Verification items for the finished model (mm, model axes). Face numbers are marked on the shaded views. A direction names the side the tool comes from. Give positions to 0.01 mm unless a question says otherwise; leave off trailing zeros. Order: outer loops, then holes, each group sorted by start corner. A loop starts at its lowest first (then second) coordinate and runs counter-clockwise, first axis right, second up. Notation, with made-up numbers: M -2,27 L 7,27 A12 cw 7,33 Z; hole C 8.25,-3 d2. An arc over 180 degrees is marked long. Answer as a JSON object with one key per item and string values.
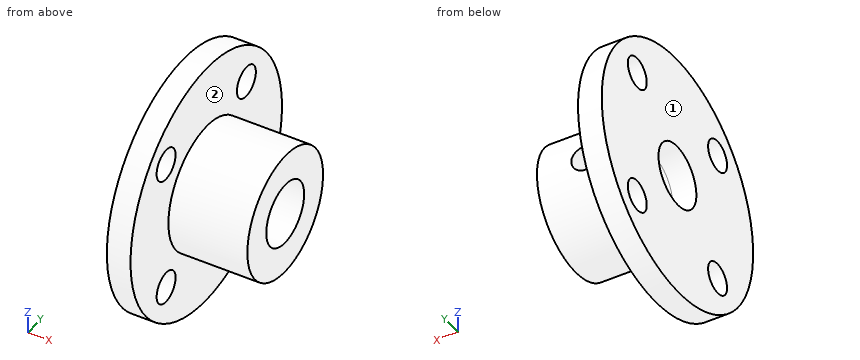
```python
from build123d import *

# Parameters (mm, degrees)
SKETCH_1_R          = 8
SKETCH_1_R_2        = 4
EXTRUDE_1_DEPTH     = 10
SKETCH_2_R          = 16
SKETCH_2_R_2        = 4
EXTRUDE_2_DEPTH     = 3
CUT_EXTRUDE_1_REACH = 5
SKETCH_3_R          = 2


with BuildPart() as part:
    # 草图1 → 凸台-拉伸1 (new body)
    with BuildSketch(Plane(origin=(0, 0, 0), x_dir=(0, 0, -1), z_dir=(1, 0, 0))):
        Circle(SKETCH_1_R)
        Circle(SKETCH_1_R_2, mode=Mode.SUBTRACT)
    extrude(amount=EXTRUDE_1_DEPTH)

    # 草图2 → 凸台-拉伸2 (add)
    with BuildSketch(Plane.ZY):
        Circle(SKETCH_2_R)
        Circle(SKETCH_2_R_2, mode=Mode.SUBTRACT)
    extrude(amount=EXTRUDE_2_DEPTH)

    # 草图3 → 切除-拉伸1 (cut, up to next)
    with BuildSketch(Plane(origin=(0, 0, 0), x_dir=(0, 0, -1), z_dir=(1, 0, 0)), mode=Mode.PRIVATE) as cut_extrude_1_sk1:
        with Locations((-8.485281374, -8.485281374)):
            Circle(SKETCH_3_R)
    cut_extrude_1_tool1 = extrude(cut_extrude_1_sk1.sketch, amount=-CUT_EXTRUDE_1_REACH, mode=Mode.PRIVATE) & part.part
    add(cut_extrude_1_tool1.solids().sort_by_distance((0, -8.485281, 8.485281))[0], mode=Mode.SUBTRACT)
    # 草图3 → 切除-拉伸1 (cut, up to next)
    with BuildSketch(Plane(origin=(0, 0, 0), x_dir=(0, 0, -1), z_dir=(1, 0, 0)), mode=Mode.PRIVATE) as cut_extrude_1_sk2:
        with Locations((8.485281374, 8.485281374)):
            Circle(SKETCH_3_R)
    cut_extrude_1_tool2 = extrude(cut_extrude_1_sk2.sketch, amount=-CUT_EXTRUDE_1_REACH, mode=Mode.PRIVATE) & part.part
    add(cut_extrude_1_tool2.solids().sort_by_distance((0, 8.485281, -8.485281))[0], mode=Mode.SUBTRACT)
    # 草图3 → 切除-拉伸1 (cut, up to next)
    with BuildSketch(Plane(origin=(0, 0, 0), x_dir=(0, 0, -1), z_dir=(1, 0, 0)), mode=Mode.PRIVATE) as cut_extrude_1_sk3:
        with Locations((-8.485281374, 8.485281374)):
            Circle(SKETCH_3_R)
    cut_extrude_1_tool3 = extrude(cut_extrude_1_sk3.sketch, amount=-CUT_EXTRUDE_1_REACH, mode=Mode.PRIVATE) & part.part
    add(cut_extrude_1_tool3.solids().sort_by_distance((0, 8.485281, 8.485281))[0], mode=Mode.SUBTRACT)
    # 草图3 → 切除-拉伸1 (cut, up to next)
    with BuildSketch(Plane(origin=(0, 0, 0), x_dir=(0, 0, -1), z_dir=(1, 0, 0)), mode=Mode.PRIVATE) as cut_extrude_1_sk4:
        with Locations((8.485281374, -8.485281374)):
            Circle(SKETCH_3_R)
    cut_extrude_1_tool4 = extrude(cut_extrude_1_sk4.sketch, amount=-CUT_EXTRUDE_1_REACH, mode=Mode.PRIVATE) & part.part
    add(cut_extrude_1_tool4.solids().sort_by_distance((0, -8.485281, -8.485281))[0], mode=Mode.SUBTRACT)

    # 草图5 → M4 螺纹孔1 (revolve, cut)
    with BuildSketch(Plane(origin=(4.000350767, 0, 0), x_dir=(0, 0, -1), z_dir=(1, 0, 0))):
        Polygon((0, 0), (0, 12.491420021), (1.65, 11.5), (1.65, 0), align=None)
    revolve(axis=Axis((4.000350767, -6.35, 0), (0, 1, 0)), mode=Mode.SUBTRACT)


solid = part.part
```
Q1. Material ranges on L1, parallel to Z at x = -1.5, y = 7.5; L2, parallel to Y at x = 7.75, z = 0; L3, parallel to Z at x = -1, y = 8.5, recorded low to high.
Resolved:
{"L1": "z = -14.13 to -10.23, -6.74 to 6.74, 10.23 to 14.13", "L2": "y = -8 to -4, 4 to 8", "L3": "z = -13.56 to -10.49, -6.49 to 6.49, 10.49 to 13.56"}
Q2. Section check D-D on z = 9.5. Record the cut outline in (x, y), then the cut area to 3 significant figures.
Resolved:
{"outline": "M -3,-12.87 L 0,-12.87 L 0,-10.21 L -3,-10.21 Z; M -3,-6.76 L 0,-6.76 L 0,6.76 L -3,6.76 Z; M -3,10.21 L 0,10.21 L 0,12.87 L -3,12.87 Z", "area": "56.6 mm²"}
Q3. Gauge pin test, flat ends, axial feed: pin 1 Ø2 at (x, y) = (8.5, -5) entering from +Z; pin 2 Ø1.5 at (x, y) = (2, -0.5) entering from -Z; pin 3 Ø2 at (x, z) = (4, 0) entering from -Y. Record the tip position at first contact, or that the pin passes through.
Resolved:
{"pin 1": "stops at z = 6.93", "pin 2": "stops at z = -8", "pin 3": "stops at y = -8"}
Q4. Section check B-B on z = 0. Record the cut outline in (x, y), then the cut area to 3 significant figures.
Resolved:
{"outline": "M -3,-16 L 0,-16 L 0,-8 L 10,-8 L 10,-4 L -3,-4 Z; M -3,4 L 2.35,4 L 2.35,8 L 0,8 L 0,16 L -3,16 Z; M 5.65,4 L 10,4 L 10,8 L 5.65,8 Z", "area": "139 mm²"}
Q5. Section check C-C on y = 0. Record the cut outline in (x, z), then the cut area to 3 significant figures.
Resolved:
{"outline": "M -3,-16 L 0,-16 L 0,-8 L 10,-8 L 10,-4 L -3,-4 Z; M -3,4 L 10,4 L 10,8 L 0,8 L 0,16 L -3,16 Z", "area": "152 mm²"}
Q6. Tool access check on the marked faces 1 and 2. Record the directions out of +Z, -Z, +X, -X, +Y, -Y that give a thin tool (end or side, any length) a straight path to the whole face; none if there is none.
Resolved:
{"face 1": "+Z, -Z, -X, +Y, -Y", "face 2": "+X"}
Q7. Section check A-A on y = -7.5. Record the cut outline in (x, z), then the cut area to 3 significant figures.
Resolved:
{"outline": "M -3,-14.13 L 0,-14.13 L 0,-10.23 L -3,-10.23 Z; M -3,-6.74 L 0,-6.74 L 0,-2.78 L 10,-2.78 L 10,2.78 L 0,2.78 L 0,6.74 L -3,6.74 Z; M -3,10.23 L 0,10.23 L 0,14.13 L -3,14.13 Z", "area": "120 mm²"}
